```python
from build123d import *

# Parameters (mm, degrees)
F2_R = 1
F3_R = 1


with BuildPart() as f1:
    # F0 (on Front) → F1 (revolve)
    with BuildSketch(Plane.XZ):
        Polygon((10.75, 49.795319), (0, 49.795319), (0, 11.795319), (0, -40.204681), (15, -40.204681), (15, 11.795319), (10.775, 11.795319), (10.775, 26.795319), (10.75, 26.795319), align=None)
    revolve(axis=Axis((0, 0, 30.795319), (0, 0, 1)))

    # F2
    f2_edges = [f1.edges().sort_by_distance(p)[0] for p in [
        (-15, 0, 11.795319),
    ]]
    fillet(f2_edges, radius=F2_R)

    # F3
    f3_edges = [f1.edges().sort_by_distance(p)[0] for p in [
        (-15, 0, -40.204681),
    ]]
    fillet(f3_edges, radius=F3_R)


solid = f1.part
```
Check sheet for the modelled part. Datum: model origin and axes. Units: mm. A direction names the side the tool comes from. Give positions to 0.01 mm unless a question says otherwise; leave off trailing zeros. Loops run counter-clockwise (first coordinate to the right, second up) from the corner with the lowest first, then second, coordinate; pieces in that order, holes last. Notation, with made-up numbers: M -14.75,69.25 L 3.25,69.25 A14 cw 3.25,77.25 Z; hole C 1.5,23 d10. An arc over 180 degrees is marked long. Answer as CSV lines item,"result".
Item 1: Sectioned sample at A-A, the plane y = 0. Enter the section's corners in (x, z) (3 decimals), then the cut area to 3 significant figures.
Reply:
outline,"M -15,-39.205 A1 ccw -14,-40.205 L 14,-40.205 A1 ccw 15,-39.205 L 15,10.795 A1 ccw 14,11.795 L 10.775,11.795 L 10.775,26.795 L 10.75,26.795 L 10.75,49.795 L -10.75,49.795 L -10.75,26.795 L -10.775,26.795 L -10.775,11.795 L -14,11.795 A1 ccw -15,10.795 Z"
area,"2,380 mm^2"
Item 2: Sectioned sample at D-D, the plane z = -23. Enter the section's corners in (x, y).
Reply:
outline,"C 0,0 d30"
Item 3: Scan lines: L1, parallel to X at y = -0.5, z = -18.5; L2, parallel to Z at x = 3, y = 12; L3, parallel to Y at x = 9, z = 46.5. Record each from-to range of solid material in increasing order.
Reply:
L1,"-14.99 to 14.99"
L2,"-40.2 to 11.8"
L3,"-5.88 to 5.88"
Item 4: Sectioned sample at C-C, the plane z = 32.5. Enter the section's corners in (x, y), then the cut area to 3 significant figures.
Reply:
outline,"C 0,0 d21.5"
area,"363 mm^2"
Item 5: Set-up check for faces 1 (the face through (0, 0, 49.795)), 2 (the face through (7.19, -8.23, 11.795)): record each of +Z, -Z, +X, -X, +Y, -Y from which the full face is reachable in a straight line by a thin tool's end or side.
Reply:
face 1,"+Z, +X, -X, +Y, -Y"
face 2,"+Z"
Item 6: Depth check by flat-ended pin: pin 1 Ø4 at (x, z) = (10, -10.5) entering from -Y; pin 2 Ø6 at (x, z) = (8.5, -14.5) entering from -Y; pin 3 Ø6 at (y, z) = (0.5, 14) entering from +X. Enter the tip coordinate at first touch or a pass-through.
Reply:
pin 1,"y = -12.69"
pin 2,"y = -13.96"
pin 3,"x = 14.97"
